The figure shows three views and two pictorial views of one solid part (mm, origin at its lowest corner). Answer the questions. Round coordinates to 2 decimals unless told otherwise and drop trailing zeros. Loops run counter-clockwise (first coordinate to the right, second up) from the corner with the lowest first, then second, coordinate; pieces in that order, holes last. Notation, with made-up numbers: (36.25, 82) -> (73.25, 82) arc R21 ccw to (73.25, 117) -> close; hole circle Ø1 at (1, 42.5). An arc over 180 degrees is marked (long way). Use a Markdown table: item, result. Add a question column.
Q1. Section B-B on z = 122 is taken. Give the vertices of the cut face in (x, y), then the cut area to 3 significant figures.
Q2. Section D-D on z = 37.5 is taken. Give the vertices of the cut face in (x, y) (1 decimal).
Q3. Section A-A on x = 163.5 is taken. Give the vertices of the cut face in (y, z).
Q4. Consider line 1 (X direction, y = 2, z = 124); line 2 (X direction, y = 3.45, z = 78); line 3 (Z direction, x = 97, y = 1.4). Determine where each line is inside the solid, lowest interval first.
Q5. Section C-C on y = 2.6 is taken. Give the number of separate pieces and of enclosed holes in the cut face, then the cut area to 3 significant figures.
Q6. Given pin 1 Ø1.2 at (x, y) = (225.5, 1.5) entering from -Z (1 decimal); pin 2 Ø6 at (x, z) = (131, 43.5) entering from -Y, each flat-ended and moving along its own axis, determine where each tip first touches the part or whether it passes through.
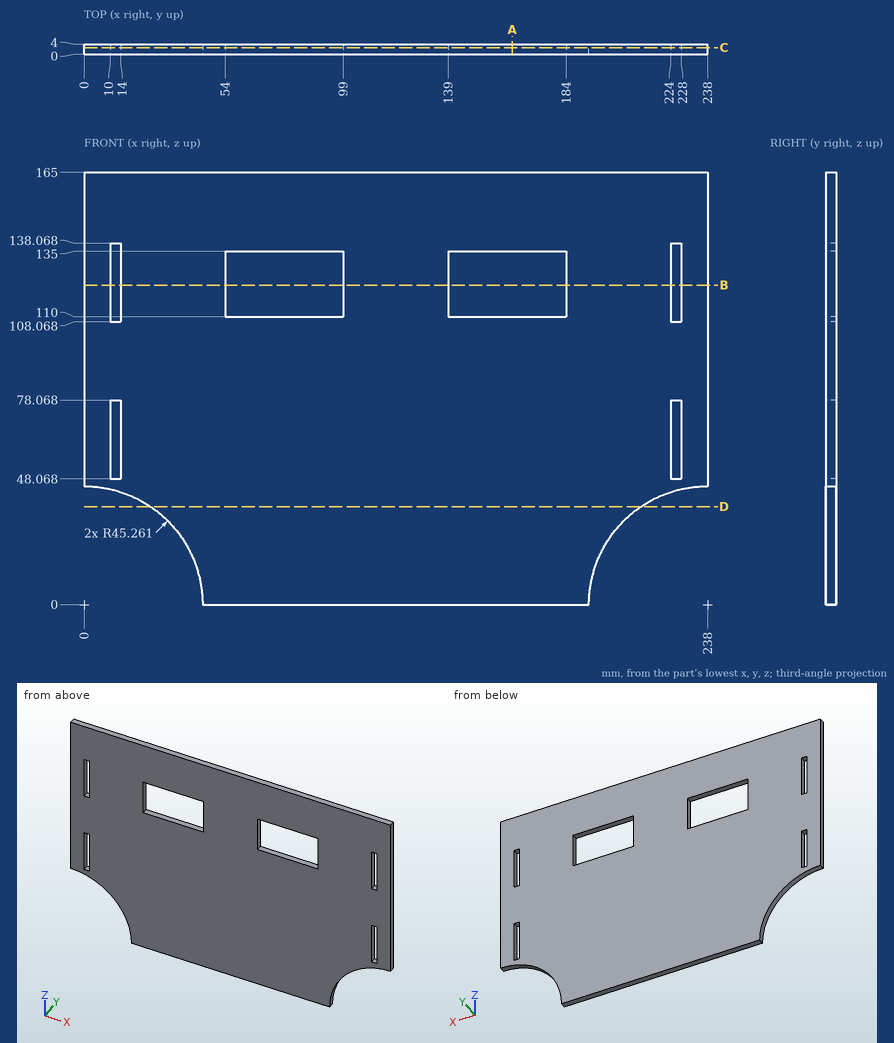
Checked values:
| question | item | result |
|---|---|---|
| 1 | outline | (0, 0) -> (10, 0) -> (10, 4) -> (0, 4) -> close; (14, 0) -> (54, 0) -> (54, 4) -> (14, 4) -> close; (99, 0) -> (139, 0) -> (139, 4) -> (99, 4) -> close; (184, 0) -> (224, 0) -> (224, 4) -> (184, 4) -> close; (228, 0) -> (238, 0) -> (238, 4) -> (228, 4) -> close |
| 1 | area | 560 mm2 |
| 2 | outline | (25.3, 0) -> (212.7, 0) -> (212.7, 4) -> (25.3, 4) -> close |
| 3 | outline | (0, 0) -> (4, 0) -> (4, 110) -> (0, 110) -> close; (0, 135) -> (4, 135) -> (4, 165) -> (0, 165) -> close |
| 4 | line 1 | x = 0 to 10, 14 to 54, 99 to 139, 184 to 224, 228 to 238 |
| 4 | line 2 | x = 0 to 10, 14 to 224, 228 to 238 |
| 4 | line 3 | z = 0 to 110, 135 to 165 |
| 5 | separate pieces | 1 |
| 5 | enclosed holes | 6 |
| 5 | area | 33,300 mm2 |
| 6 | pin 1 | stops at z = 43.3 |
| 6 | pin 2 | stops at y = 0 |
